Job drawing, mm, ordinate dimensions from the low corner. One solid piece. Round coordinates to 2 decimals unless told otherwise and drop trailing zeros. Loops run counter-clockwise (first coordinate to the right, second up) from the corner with the lowest first, then second, coordinate; pieces in that order, holes last.
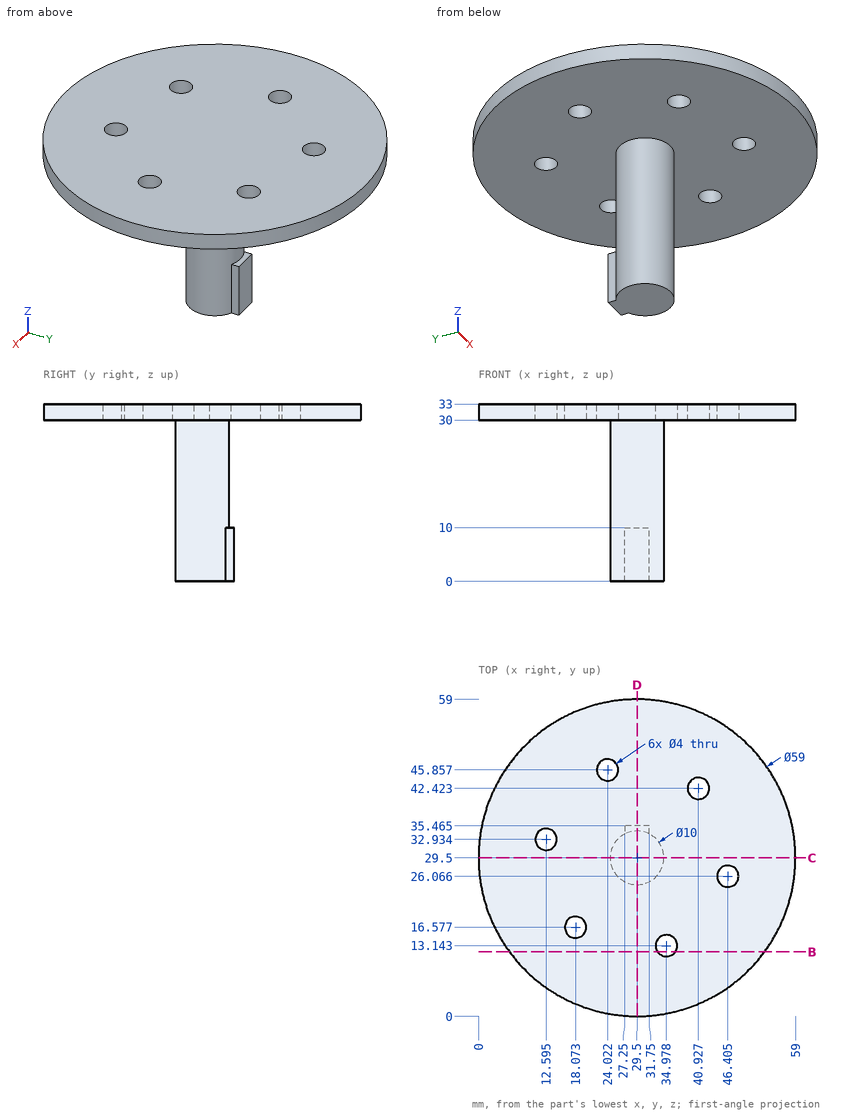
Item 1: Cut at C-C, the plane y = 29.5. Give the cut face in (x, z).
Answers follow:
outline: (0, 30) - (24.5, 30) - (24.5, 0) - (34.5, 0) - (34.5, 30) - (59, 30) - (59, 33) - (0, 33) - close
Item 2: Cut at D-D, the plane x = 29.5. Give the cut face in (y, z) (1 decimal).
Answers follow:
outline: (0, 30) - (24.5, 30) - (24.5, 0) - (35.5, 0) - (35.5, 10) - (34.5, 10) - (34.5, 30) - (59, 30) - (59, 33) - (0, 33) - close
Item 3: Cut at B-B, the plane y = 12. Give the cut face in (x, z).
Answers follow:
outline: (5.75, 30) - (33.34, 30) - (33.34, 33) - (5.75, 33) - close; (36.62, 30) - (53.25, 30) - (53.25, 33) - (36.62, 33) - close
Item 4: Flat gauge pins, fed straight in: P1, Ø3, axis at x = 24.02, y = 45.86, coming from the -Z side; P2, Ø6, axis at x = 44, y = 26.5, coming from the -Z side; P3, Ø1.2, axis at y = 34.5, z = 3.5, coming from the -X side (1 decimal); P4, Ø5, axis at x = 34.5, z = 4.5, coming from the +Y side. Where does each tip first touch, or does it go through?
Answers follow:
P1: passes through
P2: stops at z = 30
P3: stops at x = 27.1
P4: stops at y = 33.83
Item 5: Probe line 1 (X direction, y = 13.5, z = 30.5) (1 decimal); line 2 (Z direction, x = 46, y = 36); line 3 (Y direction, x = 30, z = 31) (1 decimal). List the from-to ranges inside material, lowest first.
Answers follow:
line 1: x = 4.7 to 33, 36.9 to 54.3
line 2: z = 30 to 33
line 3: y = 0 to 59
